Geometry: final body of the model. Coordinates: model frame, mm. A direction names the side the tool comes from. Give positions to 0.01 mm unless a question says otherwise; leave off trailing zeros. Loops run counter-clockwise (first coordinate to the right, second up) from the corner with the lowest first, then second, coordinate; pieces in that order, holes last. Notation, with made-up numbers: M -11.5,-33.5 L -1.5,-33.5 A23 cw -1.5,-17.5 Z; hole C -0.5,72 d3. An arc over 180 degrees is marked long. Put each result on its own line as item: value.
```python
from build123d import *

# Parameters (mm, degrees)
LOWER_HALF_CUT_DEPTH   = 58.950496115
SIDE_SHELL_CUT_1_DEPTH = 6.2
SIDE_START             = -6.2
SIDE_SHELL_CUT_2_DEPTH = 6.2
BOSS_EXTRUDE3_START    = 2.5
BOSS_EXTRUDE3_DEPTH    = 2.5
BOSS_EXTRUDE4_DEPTH    = 2.5
FILLET2_R              = 0.5


with BuildPart() as part:
    # Sketch1 → Revolve1 (revolve)
    with BuildSketch(Plane.XY, mode=Mode.PRIVATE) as revolve1_sk:
        Polygon((20.2, 0), (26.2, 0), (26.2, 17.5), (-26.2, 17.5), (-26.2, 0), (-20.2, 0), (-20.2, 15), (20.2, 15), align=None)
    revolve(revolve1_sk.sketch.rotate(Axis((0, 0, 0), (-1, 0, 0)), 90), axis=Axis((0, 0, 0), (-1, 0, 0)))

    # Sketch2 → lower half cut (cut, through all)
    with BuildSketch(Plane.ZY.offset(26.2)):
        with BuildLine():
            Line((-17.5, 0), (17.5, 0))
            ThreePointArc((17.5, 0), (0, -17.5), (-17.5, 0))
        make_face()
    extrude(amount=-LOWER_HALF_CUT_DEPTH, mode=Mode.SUBTRACT)

    # Sketch3 → side shell cut 1 (cut)
    with BuildSketch(Plane.ZY.offset(26.2)):
        with BuildLine():
            Line((-17.5, 0), (17.5, 0))
            ThreePointArc((17.5, 0), (15.483862567, 8.154753215), (9.9, 14.430523206))
            Line((9.9, 14.430523206), (9.9, 11.861406616))
            Line((9.9, 11.861406616), (-9.9, 11.861406616))
            Line((-9.9, 11.861406616), (-9.9, 14.430523206))
            ThreePointArc((-9.9, 14.430523206), (-15.483862567, 8.154753215), (-17.5, 0))
        make_face()
    extrude(amount=-SIDE_SHELL_CUT_1_DEPTH, mode=Mode.SUBTRACT)

    # Sketch4 → side shell cut 2 (cut)
    with BuildSketch(Plane(origin=(26.2, 0, 0), x_dir=(0, 0, -1), z_dir=(1, 0, 0)).offset(SIDE_START)):
        with BuildLine():
            Line((-17.5, 0), (17.5, 0))
            ThreePointArc((17.5, 0), (15.483862567, 8.154753215), (9.9, 14.430523206))
            Line((9.9, 14.430523206), (9.9, 11.861406616))
            Line((9.9, 11.861406616), (-9.9, 11.861406616))
            Line((-9.9, 11.861406616), (-9.9, 14.430523206))
            ThreePointArc((-9.9, 14.430523206), (-15.483862567, 8.154753215), (-17.5, 0))
        make_face()
    extrude(amount=SIDE_SHELL_CUT_2_DEPTH, mode=Mode.SUBTRACT)

    # Sketch5 → Boss-Extrude3 (add)
    with BuildSketch(Plane.ZY.offset(26.2).offset(BOSS_EXTRUDE3_START)):
        with BuildLine():
            Line((-9.9, 14.430523206), (-9.9, 11.861406616))
            Line((-9.9, 11.861406616), (-9.9, 6.861406616))
            Line((-9.9, 6.861406616), (9.9, 6.861406616))
            Line((9.9, 6.861406616), (9.9, 11.861406616))
            Line((9.9, 11.861406616), (9.9, 14.430523206))
            ThreePointArc((9.9, 14.430523206), (0, 17.5), (-9.9, 14.430523206))
        make_face()
    extrude(amount=-BOSS_EXTRUDE3_DEPTH)

    # Sketch7 → Boss-Extrude4 (add)
    with BuildSketch(Plane(origin=(26.2, 0, 0), x_dir=(0, 0, -1), z_dir=(1, 0, 0))):
        with BuildLine():
            Line((-9.9, 6.861406616), (9.9, 6.861406616))
            Line((9.9, 6.861406616), (9.9, 14.430523206))
            ThreePointArc((9.9, 14.430523206), (0, 17.5), (-9.9, 14.430523206))
            Line((-9.9, 14.430523206), (-9.9, 6.861406616))
        make_face()
    extrude(amount=BOSS_EXTRUDE4_DEPTH)

    # Fillet2
    fillet2_edges = [part.edges().sort_by_distance(p)[0] for p in [
        (27.45, 6.861406616, -9.9),
        (27.45, 6.861406616, 9.9),
        (28.7, 10.645964911, -9.9),
        (28.7, 17.5, 0),
        (28.7, 10.645964911, 9.9),
        (28.7, 6.861406616, 0),
        (-27.45, 6.861406616, -9.9),
        (-27.45, 6.861406616, 9.9),
        (-28.7, 6.861406616, 0),
        (-28.7, 10.645964911, 9.9),
        (-28.7, 17.5, 0),
        (-28.7, 10.645964911, -9.9),
    ]]
    fillet(fillet2_edges, radius=FILLET2_R)


solid = part.part
```
Item 1: Pin query (flat end, axial travel): pin 1 Ø1 at (x, z) = (-27.5, -2) entering from -Y; pin 2 Ø2 at (x, y) = (22.5, 12.5) entering from +Z; pin 3 Ø6 at (x, y) = (2, 12) entering from +Z. Return the tip coordinate at first contact, or that it passes through.
Output values:
pin 1: y = 6.86
pin 2: z = 9.9
pin 3: z = 15.01
Item 2: Section A-A on z = 0. Output: boundary loops of the cut face in (x, y), then the cut area to 3 significant figures.
Output values:
outline: M -28.7,7.36 A0.5 ccw -28.2,6.86 L -26.2,6.86 L -26.2,11.86 L -20.2,11.86 L -20.2,15 L 20.2,15 L 20.2,11.86 L 26.2,11.86 L 26.2,6.86 L 28.2,6.86 A0.5 ccw 28.7,7.36 L 28.7,17 A0.5 ccw 28.2,17.5 L -28.2,17.5 A0.5 ccw -28.7,17 Z
area: 222 mm²
Item 3: Mould query, pull axis Z, two halves, no side actions, for faces 1 (the flat face through (-28.7, 12, 0)), 2 (the flat face through (-20.2, 13, 0)), 3 (the flat face through (25, 13, 9.9)). Classes: pulls with the +Z half, pulls with the -Z half, needs draft (parallel to the pull), parting line crosses it, or undercut.
Output values:
face 1: needs draft
face 2: undercut
face 3: pulls with the +Z half
Item 4: Section C-C on y = 13.5. Output: boundary loops of the cut face in (x, z), then the cut area to 3 significant figures.
Output values:
outline: M -28.7,-9.4 A0.5 ccw -28.2,-9.9 L -20,-9.9 L -20,-11.14 L 20,-11.14 L 20,-9.9 L 28.2,-9.9 A0.5 ccw 28.7,-9.4 L 28.7,9.4 A0.5 ccw 28.2,9.9 L 20,9.9 L 20,11.14 L -20,11.14 L -20,9.9 L -28.2,9.9 A0.5 ccw -28.7,9.4 Z; hole M -20.2,-6.54 L 20.2,-6.54 L 20.2,6.54 L -20.2,6.54 Z
area: 707 mm²
Item 5: Line query: probe 1 along X at (y, z) = (8.25, 5.5); probe 2 along X at (y, z) = (12.75, -2.5); probe 3 along Z at (x, y) = (16, 6.5). Output: solid intervals per line, ascending. Write a range as [from, to].
Output values:
probe 1: [-28.7, -26.2], [26.2, 28.7]
probe 2: [-28.7, -20.2], [20.2, 28.7]
probe 3: [-16.25, -13.52], [13.52, 16.25]
Item 6: Set-up query: faces 4 (the flat face through (23, 11.861, 0)), 5 (the flat face through (-25.1, 12.4, 9.9)), 6 (the flat face through (20.2, 13, 0)). Return all of +Z, -Z, +X, -X, +Y, -Y with unobstructed straight access to the full face (end or side cutting, diameter ignored); none if empty.
Output values:
face 4: +Z, -Z, -Y
face 5: +Z, -X, +Y, -Y
face 6: -Y
Item 7: Section D-D on x = 17.5. Output: boundary loops of the cut face in (y, z), then the cut area to 3 significant figures.
Output values:
outline: M 0,-17.5 A17.5 ccw 0,17.5 L 0,15 A15 cw 0,-15 Z
area: 128 mm²
Item 8: Section B-B on y = 10.75. Output: boundary loops of the cut face in (x, z), then the cut area to 3 significant figures.
Output values:
outline: M -28.7,-9.4 A0.5 ccw -28.2,-9.9 L -26.2,-9.9 L -26.2,9.9 L -28.2,9.9 A0.5 ccw -28.7,9.4 Z; M -20,-13.81 L 20,-13.81 L 20,-10.46 L -20,-10.46 Z; M -20,10.46 L 20,10.46 L 20,13.81 L -20,13.81 Z; M 26.2,-9.9 L 28.2,-9.9 A0.5 ccw 28.7,-9.4 L 28.7,9.4 A0.5 ccw 28.2,9.9 L 26.2,9.9 Z
area: 367 mm²
